Autodesk Inventor part; units mm, degrees
ref_plane "YZ Plane" through (0, 0, 0) normal (1, 0, 0) x (0, 1, 0)
ref_plane "XZ Plane" through (0, 0, 0) normal (0, 1, 0) x (-1, 0, 0)
ref_plane "XY Plane" through (0, 0, 0) normal (0, 0, 1) x (1, 0, 0)
sketch "Sketch1" plane through (0, 0, 0) normal (0, 0, 1) x (1, 0, 0)
  line L0 (-40.5, 20) -> (40.5, 20)
  line L1 (40.5, 20) -> (40.5, -20)
  line L2 (40.5, -20) -> (-40.5, -20)
  line L3 (-40.5, -20) -> (-40.5, 20)
  point P0 (0, 0)
  dimension "d0" = 81
  dimension "d1" = 40
  dimension "d2" = 20
  dimension "d3" = 40.5
extrude "Extrusion1" add sketch "Sketch1" along normal blind 1
sketch "Sketch2" plane through (0, 0, 1) normal (0, 0, 1) x (1, 0, 0)
  line L0 (40.5, 20) -> (-40.5, 20)
  line L1 (-21.8, 20) -> (-11.7, 20)
  line L2 (-11.7, 20) -> (-11.7, 16.1)
  line L3 (-11.7, 16.1) -> (-21.8, 16.1)
  line L4 (-21.8, 16.1) -> (-21.8, 20)
  line L5 (-40.5, 20) -> (-40.5, -20)
  point P0 (0, 0)
  dimension "d6" = 18.7
  dimension "d7" = 28.8
  dimension "d8" = 3.9
extrude "Extrusion2" cut sketch "Sketch2" against normal blind 1
chamfer "Chamfer1" distance 3.88 angle 45 2 edges at (-21.8, 20, 0.5) (-11.7, 20, 0.5)
sketch "Sketch3" plane through (0, 0, 1) normal (0, 0, 1) x (1, 0, 0)
  line L0 (-25.68, 20) -> (-40.5, 20)
  line L1 (-35.04, 20) -> (-25.77, 20)
  line L2 (-25.77, 20) -> (-25.77, 12.38)
  line L3 (-25.77, 12.38) -> (-35.04, 12.38)
  line L4 (-35.04, 12.38) -> (-35.04, 20)
  line L5 (-40.5, 20) -> (-40.5, -20)
  point P0 (0, 0)
  dimension "d14" = 5.46
  dimension "d15" = 14.73
  dimension "d16" = 7.62
extrude "Extrusion3" add sketch "Sketch3" along normal blind 3.2
fillet "Fillet1" radius 2 2 edges at (-35.04, 16.19, 4.2) (-25.77, 16.19, 4.2)
sketch "Sketch4" plane through (0, 0, 1) normal (0, 0, 1) x (1, 0, 0)
  line L0 (-11.7, 16.1) -> (-21.8, 16.1)
  line L1 (-21.8, 16.1) -> (-11.8, 16.1)
  line L2 (-11.8, 16.1) -> (-11.8, 12.3)
  line L3 (-11.8, 12.3) -> (-21.8, 12.3)
  line L4 (-21.8, 12.3) -> (-21.8, 16.1)
  point P0 (0, 0)
  dimension "d20" = 3.8
  dimension "d21" = 10
extrude "Extrusion4" add sketch "Sketch4" along normal blind 3.2
sketch "Sketch5" plane through (-21.8, 16.1, 0) normal (0, 1, 0) x (1, 0, 0)
  line L0 (1.2, -3.6) -> (3.4, -3.6)
  line L1 (3.4, -3.6) -> (3.4, -1.2)
  line L2 (3.4, -1.2) -> (1.2, -1.2)
  line L3 (1.2, -1.2) -> (1.2, -3.6)
  line L4 (10, -4.2) -> (0, -4.2)
  line L5 (0, -1) -> (0, -4.2)
  point P0 (21.8, 0)
  dimension "d24" = 0.6
  dimension "d25" = 1.2
  dimension "d26" = 2.4
  dimension "d27" = 2.2
extrude "Extrusion5" add sketch "Sketch5" along normal blind 2.8
sketch "Sketch6" plane through (0, 0, 1) normal (0, 0, 1) x (1, 0, 0)
  line L0 (-40.5, 20) -> (-40.5, -20)
  line L1 (-40.5, -20) -> (40.5, -20)
  point P0 (0, 0)
  point P1 (-37.5, -17)
  point P2 (-12.5, -17)
  point P3 (12.5, -17)
  point P4 (37.5, -17)
  dimension "d30" = 3
  dimension "d31" = 28
  dimension "d32" = 53
  dimension "d33" = 78
  dimension "d34" = 3
  dimension "d35" = 3
  dimension "d36" = 3
  dimension "d37" = 3
hole "Hole1" at (-37.5, -17, 1) at (-12.5, -17, 1) at (12.5, -17, 1) at (37.5, -17, 1) direction (0, 0, -1) diameter 2 depth 4 tip angle 118
sketch "Sketch7" plane through (0, 0, 1) normal (0, 0, 1) x (1, 0, 0)
  line L0 (-40.5, 20) -> (-40.5, -20)
  line L1 (-40.5, -20) -> (40.5, -20)
  point P0 (0, 0)
  point P1 (-37.5, 17)
  point P2 (37.5, 17)
  dimension "d45" = 3
  dimension "d46" = 37
  dimension "d47" = 78
  dimension "d48" = 37
hole "Hole2" at (-37.5, 17, 1) at (37.5, 17, 1) direction (0, 0, -1) diameter 2 depth 4 tip angle 118
sketch "Sketch8" plane through (0, 0, 1) normal (0, 0, 1) x (1, 0, 0)
  line L0 (-40.5, -20) -> (40.5, -20)
  line L1 (17.5, -20) -> (32.5, -20)
  line L2 (32.5, -20) -> (32.5, -17.3)
  line L3 (32.5, -17.3) -> (17.5, -17.3)
  line L4 (17.5, -17.3) -> (17.5, -20)
  line L5 (-40.5, 20) -> (-40.5, -20)
  point P0 (0, 0)
  dimension "d56" = 58
  dimension "d57" = 73
  dimension "d58" = 2.7
extrude "Extrusion6" cut sketch "Sketch8" against normal blind 2
chamfer "Chamfer2" distance 2.7 angle 45 2 edges at (17.5, -20, 0.5) (32.5, -20, 0.5)
sketch "Sketch9" plane through (0, 0, 1) normal (0, 0, 1) x (1, 0, 0)
  line L0 (-39.36, 4.4) -> (-33.5, 4.4)
  line L1 (-33.5, 4.4) -> (-33.5, -3.1)
  line L2 (-33.5, -3.1) -> (-39.36, -3.1)
  line L3 (-39.36, -3.1) -> (-39.36, 4.4)
  line L4 (-40.5, 20) -> (-40.5, -20)
  line L5 (-40.5, -20) -> (14.8, -20)
  line L6 (-38.86, 3.9) -> (-34, 3.9)
  line L7 (-34, 3.9) -> (-34, -2.6)
  line L8 (-34, -2.6) -> (-38.86, -2.6)
  line L9 (-38.86, -2.6) -> (-38.86, 3.9)
  line L10 (-39.36, 2.7) -> (-38.86, 2.7)
  line L11 (-38.86, 2.7) -> (-38.86, -1.4)
  line L12 (-38.86, -1.4) -> (-39.36, -1.4)
  line L13 (-39.36, -1.4) -> (-39.36, 2.7)
  point P0 (0, 0)
  dimension "d64" = 1.14
  dimension "d65" = 7
  dimension "d66" = 16.9
  dimension "d67" = 24.4
  dimension "d68" = 0.5
  dimension "d69" = 0.5
  dimension "d70" = 0.5
  dimension "d71" = 0.5
  dimension "d72" = 1.2
  dimension "d73" = 1.2
extrude "Extrusion7" add sketch "Sketch9" along normal blind 7 contours L0 L1 L2 L3 L12 L9 L8 L7 L6 L10
sketch "Sketch10" plane through (0, 0, 1) normal (0, 0, 1) x (1, 0, 0)
  line L0 (-36.9032, 2.5042) -> (-36.1235, 2.5042)
  line L1 (-36.1235, 2.5042) -> (-36.1235, 2.0109)
  line L2 (-36.1235, 2.0109) -> (-36.9032, 2.0109)
  line L3 (-36.9032, 2.0109) -> (-36.9032, 2.5042)
  line L4 (-36.9032, -0.8534) -> (-36.1235, -0.8534)
  line L5 (-36.1235, -0.8534) -> (-36.1235, -1.3626)
  line L6 (-36.1235, -1.3626) -> (-36.9032, -1.3626)
  line L7 (-36.9032, -1.3626) -> (-36.9032, -0.8534)
  point P0 (0, 0)
extrude "Extrusion8" add sketch "Sketch10" along normal blind 5
sketch "Sketch11" plane through (0, 0, 1) normal (0, 0, 1) x (1, 0, 0)
  line L0 (40.5, -20) -> (40.5, 20)
  line L1 (40.5, 11) -> (14.5, 11)
  line L2 (14.5, 11) -> (14.5, -7.2)
  line L3 (14.5, -7.2) -> (40.5, -7.2)
  line L4 (40.5, -7.2) -> (40.5, 11)
  line L5 (-40.5, 20) -> (-40.5, -20)
  line L6 (40.5, 20) -> (-7.82, 20)
  point P0 (0, 0)
  dimension "d78" = 55
  dimension "d79" = 9
  dimension "d80" = 18.2
extrude "Extrusion9" add sketch "Sketch11" along normal blind 1
sketch "Sketch12" plane through (0, 0, 2) normal (0, 0, 1) x (1, 0, 0)
  line L0 (16.5, 9) -> (34, 9)
  line L1 (34, 9) -> (34, -5.2)
  line L2 (34, -5.2) -> (16.5, -5.2)
  line L3 (16.5, -5.2) -> (16.5, 9)
  line L4 (40.5, 11) -> (14.5, 11)
  line L5 (14.5, -7.2) -> (40.5, -7.2)
  line L6 (14.5, 11) -> (14.5, -7.2)
  line L7 (40.5, -7.2) -> (40.5, 11)
  point P0 (0, 0)
  dimension "d83" = 2
  dimension "d84" = 2
  dimension "d85" = 2
  dimension "d86" = 6.5
extrude "Extrusion10" add sketch "Sketch12" along normal blind 3 contours L0 L1 L2 L3
fillet "Fillet2" radius 0.5 4 edges at (25.25, 9, 5) (16.5, 1.9, 5) (25.25, -5.2, 5) (34, 1.9, 5)
sketch "Sketch13" plane through (0, 0, 0) normal (0, 0, -1) x (-1, 0, 0)
  line L0 (-4.4, -16.1) -> (4.4, -16.1)
  line L1 (4.4, -16.1) -> (4.4, -19.4)
  line L2 (4.4, -19.4) -> (-4.4, -19.4)
  line L3 (-4.4, -19.4) -> (-4.4, -16.1)
  line L4 (40.5, 20) -> (40.5, -20)
  line L5 (40.5, -20) -> (-14.8, -20)
  point P0 (0, 0)
  dimension "d90" = 36.1
  dimension "d91" = 44.9
  dimension "d92" = 0.6
  dimension "d93" = 3.9
extrude "Extrusion11" add sketch "Sketch13" along normal blind 6
fillet "Fillet3" radius 1.28 4 edges at (4.4, -16.1, -3) (4.4, -19.4, -3) (-4.4, -16.1, -3) (-4.4, -19.4, -3)
sketch "Sketch14" plane through (0, 0, 0) normal (0, 0, -1) x (-1, 0, 0)
  line L0 (-32.5, -2.3) -> (-17.3, -2.3)
  line L1 (-17.3, -2.3) -> (-17.3, -17.3)
  line L2 (-17.3, -17.3) -> (-32.5, -17.3)
  line L3 (-32.5, -17.3) -> (-32.5, -2.3)
  line L4 (40.5, 20) -> (40.5, -20)
  line L5 (-32.5, -17.3) -> (-17.5, -17.3)
  point P0 (0, 0)
  dimension "d97" = 57.8
  dimension "d98" = 73
  dimension "d99" = 15
extrude "Extrusion12" add sketch "Sketch14" along normal blind 2.2
properties part number "mcu-unit"
The model under review builds one solid part; all positions refer to its coordinate system, in mm. A direction names the side the tool comes from. Round coordinates to 2 decimals unless told otherwise and drop trailing zeros. Write each loop counter-clockwise with the first axis right and the second up, starting at its lowest first coordinate (ties: lowest second). Pieces come first, ordered by that corner, then holes. Notation, with made-up numbers: (34.5, 77.5) - (56.5, 77.5) arc R26 ccw to (56.5, 108.5) - close; hole circle Ø7 at (61, 18.5). An arc over 180 degrees is marked (long way). One line per question, with ' | ' between items.
Item 1: Add section C-C, the plane y = -13.5. Give the boundary of the cut face in (x, z), then the cut area to 3 significant figures.
Resolved:
outline: (-40.5, 0) - (17.3, 0) - (17.3, -2.2) - (32.5, -2.2) - (32.5, 0) - (40.5, 0) - (40.5, 1) - (-40.5, 1) - close | area: 114 mm2
Item 2: To check wall thickness, follow probe 1 along Y at (x, z) = (37.5, 0.25); probe 2 along Y at (x, z) = (-12.5, 0.6); probe 3 along Y at (x, z) = (12.5, 0.35). State the ranges of each line that lie inside material, in increasing order.
Resolved:
probe 1: y = -20 to -18, -16 to 16, 18 to 20 | probe 2: y = -20 to -18, -16 to 16.1 | probe 3: y = -20 to -18, -16 to 20
Item 3: For P1, Ø1, axis at x = -21, y = 5.5, coming from the -Z side; P2, Ø2, axis at x = -22, y = 7.5, coming from the +Z side; P3, Ø2.5, axis at x = -36, z = 4, coming from the +Y side, all flat-tipped, find the tip position at first contact; note any pin that passes through.
Resolved:
P1: stops at z = 0 | P2: stops at z = 1 | P3: stops at y = 4.4
Item 4: The part is to be moulded in two halves that separate along X. For faces 1 (the face through (-20, 17, 3.6)), 2 (the face through (-18.4, 17, 2)), 3 (the face through (36.66, 16.46, 0.49)), say which applies: pulls with the +X half, pulls with the -X half, needs draft (parallel to the pull), parting line crosses it, or undercut.
Resolved:
face 1: needs draft | face 2: pulls with the +X half | face 3: undercut
Item 5: Add section D-D, the plane y = 17. Give the boundary of the cut face in (x, z), then the cut area to 3 significant figures.
Resolved:
outline: (-40.5, 0) - (-38.5, 0) - (-38.5, 1) - (-40.5, 1) - close; (-36.5, 0) - (-22.68, 0) - (-22.68, 1) - (-25.77, 1) - (-25.77, 2.2) arc R2 ccw to (-27.77, 4.2) - (-33.04, 4.2) arc R2 ccw to (-35.04, 2.2) - (-35.04, 1) - (-36.5, 1) - close; (-20.6, 1.2) - (-18.4, 1.2) - (-18.4, 3.6) - (-20.6, 3.6) - close; (-10.82, 0) - (36.5, 0) - (36.5, 1) - (-10.82, 1) - close; (38.5, 0) - (40.5, 0) - (40.5, 1) - (38.5, 1) - close | area: 98.4 mm2
Item 6: Add section A-A, the plane z = -1.25. Give the boundary of the cut face in (x, y), then the cut area to 3 significant figures.
Resolved:
outline: (-4.4, -18.12) arc R1.28 ccw to (-3.12, -19.4) - (3.12, -19.4) arc R1.28 ccw to (4.4, -18.12) - (4.4, -17.38) arc R1.28 ccw to (3.12, -16.1) - (-3.12, -16.1) arc R1.28 ccw to (-4.4, -17.38) - close; (17.3, -17.3) - (32.5, -17.3) - (32.5, -2.3) - (17.3, -2.3) - close | area: 256 mm2
Item 7: For faces 4 (the face through (16.1, -18.7, 0.5)), 5 (the face through (25, -2.3, -1)), 6 (the face through (0, -19.4, -3)), 7 (the face through (-20.6, 17, 2)), 8 (the face through (-21.8, 14, 3)), list the 3-axis set-ups (+Z, -Z, +X, -X, +Y, -Y) from which the entire face can be reached by the end or side of a thin tool; tool diameter is ignored.
Resolved:
face 4: +Z, -Z, -Y | face 5: -Z, +X, -X, +Y | face 6: -Z, +X, -X, -Y | face 7: +Z, -Z, +Y | face 8: +Z, +Y, -Y
Item 8: Add section B-B, the plane x = 12.5. Give the boundary of the cut face in (y, z), then the cut area to 3 significant figures.
Resolved:
outline: (-20, 0) - (-18, 0) - (-18, 1) - (-20, 1) - close; (-16, 0) - (20, 0) - (20, 1) - (-16, 1) - close | area: 38.0 mm2
